from build123d import *

# Parameters (mm, degrees)
SKETCH_1_W      = 12
SKETCH_1_H      = 17
EXTRUDE_1_DEPTH = 11
SKETCH_2_W      = 15
SKETCH_2_H      = 21
EXTRUDE_2_DEPTH = 2
CHAMFER_1_SIZE  = 2
EXTRUDE_3_DEPTH = 4.5


with BuildPart() as part:
    # 草图1 → 凸台-拉伸1 (new body)
    with BuildSketch(Plane(origin=(0, 0, 0), x_dir=(1, 0, 0), z_dir=(0, 1, 0))):
        Rectangle(SKETCH_1_W, SKETCH_1_H)
    extrude(amount=EXTRUDE_1_DEPTH)

    # 草图2 → 凸台-拉伸2 (add)
    with BuildSketch(Plane(origin=(0, 11, 0), x_dir=(1, 0, 0), z_dir=(0, 1, 0))):
        Rectangle(SKETCH_2_W, SKETCH_2_H)
    extrude(amount=EXTRUDE_2_DEPTH)

    # 倒角1
    chamfer_1_edges = [part.edges().sort_by_distance(p)[0] for p in [
        (0, 13, -10.5),
        (7.5, 13, 0),
        (0, 13, 10.5),
        (-7.5, 13, 0),
    ]]
    chamfer(chamfer_1_edges, length=CHAMFER_1_SIZE - 0.0001)  # a hair under: the kernel refuses the full size

    # 草图3 → 凸台-拉伸3 (add, symmetric)
    with BuildSketch(Plane(origin=(0, 0, 0), x_dir=(0, 0, -1), z_dir=(1, 0, 0))):
        Polygon((-6.993584735, 13), (-4.673908178, 16.758295881), (0, 13), align=None)
    extrude(amount=EXTRUDE_3_DEPTH, both=True)


solid = part.part
Can you work these out from the model? Positions are in its coordinate system, mm. A direction names the side the tool comes from. Give positions to 0.01 mm unless a question says otherwise; leave off trailing zeros. Loops run counter-clockwise (first coordinate to the right, second up) from the corner with the lowest first, then second, coordinate; pieces in that order, holes last. Notation, with made-up numbers: (-25, 3) - (-21, 3) arc R20 cw to (-21, 31) - close; hole circle Ø7 at (-12.5, -16.5). An arc over 180 degrees is marked (long way). One line per item, written item: value.
(1) I'm going to push flat-ended pins straight in: pin 1 (3 mm diameter, centred on x = 0, z = 6.5, fed in from +Y); pin 2 (1.5 mm diameter, centred on x = 0, y = 6.5, fed in from -Z); pin 3 (4 mm diameter, centred on x = 0.5, y = 4.5, fed in from +Z). Where does each tip first touch, or does it pass through?
Verdict:
pin 1: y = 16.23
pin 2: z = -8.5
pin 3: z = 8.5
(2) I need wall thicknesses on line 1 along X through (y, z) = (3.75, -1); line 2 along Z through (x, y) = (-2, 10.5); line 3 along Y through (x, z) = (-2.75, -5). Which ranges of each line are inside material? Lowest first, please.
Verdict:
line 1: -6 to 6
line 2: -8.5 to 8.5
line 3: 0 to 13
(3) On a 3-axis mill with a long thin cutter (end or side, diameter ignored), from which of +Z, -Z, +X, -X, +Y, -Y can I reach the whole of each face in a straight line? I mean faces 1 (the face through (0, 5, 8.5)), 2 (the face through (4.5, 14, 4)), 3 (the face through (-4.5, 14, 4)), 4 (the face through (0, 5, -8.5)). Say none if no direction works.
Verdict:
face 1: +Z, +X, -X, -Y
face 2: +Z, -Z, +X, +Y
face 3: +Z, -Z, -X, +Y
face 4: -Z, +X, -X, -Y
(4) If we section it at C-C, the plane y = 4.25: List the corners of the cut face in (x, z) for me, plus the area to 3 significant figures.
Verdict:
outline: (-6, -8.5) - (6, -8.5) - (6, 8.5) - (-6, 8.5) - close
area: 204 mm^2
